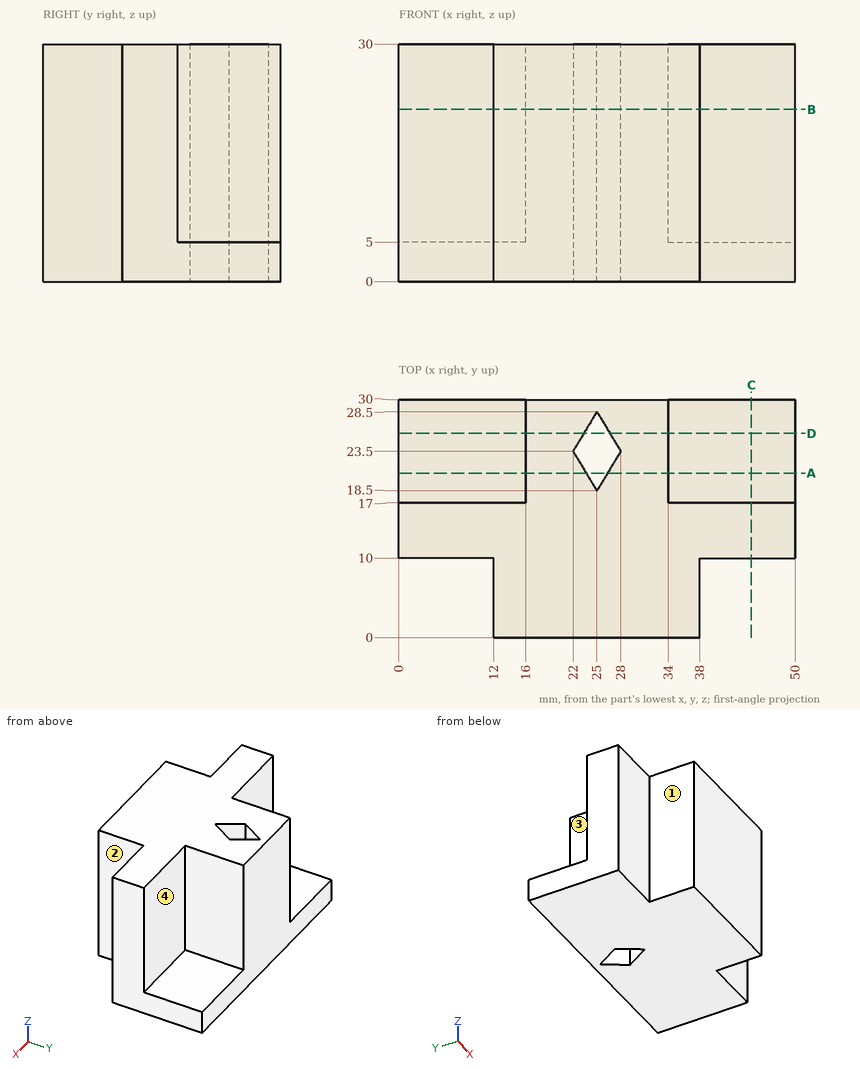
Study the drawing (mm; zero at the part's minimum x, y, z) and answer. A direction names the side the tool comes from. Round coordinates to 2 decimals unless told otherwise and drop trailing zeros. Write each loop counter-clockwise with the first axis right and the second up, starting at its lowest first coordinate (ties: lowest second). Pieces come first, ordered by that corner, then holes. Notation, with made-up numbers: (50.5, 22.5) -> (93.5, 22.5) arc R19 ccw to (93.5, 58.5) -> close; hole circle Ø1 at (74.25, 43.5). An arc over 180 degrees is marked (long way). Write each question's results on one line, items separated by ' | '.
Item 1: Find the intervals of material crossed by line 1 along Y through (x, z) = (44.5, 28.25); line 2 along X through (y, z) = (5.25, 15.75); line 3 along Y through (x, z) = (37.5, 15.5), in increasing order. Write a range as [from, to].
Result set:
line 1: [10, 17] | line 2: [12, 38] | line 3: [0, 17]
Item 2: A cutting plane is placed at A-A, the plane y = 20.75. Determine the outline of the cut face in (x, z), plus the area to 3 significant figures.
Result set:
outline: (0, 0) -> (23.65, 0) -> (23.65, 30) -> (16, 30) -> (16, 5) -> (0, 5) -> close; (26.35, 0) -> (50, 0) -> (50, 5) -> (34, 5) -> (34, 30) -> (26.35, 30) -> close | area: 619 mm^2
Item 3: A cutting plane is placed at D-D, the plane y = 25.75. Determine the outline of the cut face in (x, z).
Result set:
outline: (0, 0) -> (23.35, 0) -> (23.35, 30) -> (16, 30) -> (16, 5) -> (0, 5) -> close; (26.65, 0) -> (50, 0) -> (50, 5) -> (34, 5) -> (34, 30) -> (26.65, 30) -> close
Item 4: Flat-ended cylindrical pins translate along their axes: P1, Ø6.5, axis at y = 24, z = 20.5, coming from the +X side; P2, Ø3, axis at y = 3.5, z = 15.5, coming from the +X side; P3, Ø9.5, axis at x = 5, z = 15.5, coming from the -Y side. Find the tip coordinate at first contact, or state that the pin passes through.
Result set:
P1: x = 34 | P2: x = 38 | P3: y = 10
Item 5: A cutting plane is placed at B-B, the plane z = 21.75. Determine the outline of the cut face in (x, y), plus the area to 3 significant figures.
Result set:
outline: (0, 10) -> (12, 10) -> (12, 0) -> (38, 0) -> (38, 10) -> (50, 10) -> (50, 17) -> (34, 17) -> (34, 30) -> (16, 30) -> (16, 17) -> (0, 17) -> close; hole (22, 23.5) -> (25, 18.5) -> (28, 23.5) -> (25, 28.5) -> close | area: 814 mm^2
Item 6: Which of the six approach directions +Z, -Z, +X, -X, +Y, -Y give full straight-line access (tool end or side, diameter ignored) to the marked faces 1, 2, 3 and 4?
Result set:
face 1: +Z, -Z, -X, -Y | face 2: +Z, -Z, +X, -Y | face 3: +Z, -X, +Y | face 4: +Z, +X, +Y
Item 7: A cutting plane is placed at C-C, the plane x = 44.5. Determine the outline of the cut face in (y, z).
Result set:
outline: (10, 0) -> (30, 0) -> (30, 5) -> (17, 5) -> (17, 30) -> (10, 30) -> close
